Geometry check sheet. Reference: the model listing, model coordinates, mm. A direction names the side the tool comes from. Give positions to 0.01 mm unless a question says otherwise; leave off trailing zeros. Loops run counter-clockwise (first coordinate to the right, second up) from the corner with the lowest first, then second, coordinate; pieces in that order, holes last. Notation, with made-up numbers: (-31, 62) -> (-26, 62) arc R11 ccw to (-26, 72) -> close; hole circle Ø1 at (58, -30.75). An arc over 180 degrees is marked (long way). Write each question's results on one line, items separated by ' | '. Start each with the question number.
1) Set-up check for faces 1 (the face through (-33, 2, -5.1)), 2 (the face through (-41.133, 1.479, -1.286)), 3 (the face through (31, 2, 9)), 4 (the face through (19, 1, -6)), 5 (the face through (21, 1, 6)): record each of +Z, -Z, +X, -X, +Y, -Y from which the full face is reachable in a straight line by a thin tool's end or side.
2) Draft check along X on faces 6 (the face through (1, 0, -5)), 7 (the face through (-27.574, 1.521, -11.238)), 8 (the face through (17.5, 1.5, 5)), 9 (the face through (-41.5, 2, -7)). Enter one of: pulls with the +X half, pulls with the -X half, needs draft (parallel to the pull), parting line crosses it, or undercut.
3) Scan lines: line 1 (X direction, y = 1.6, z = 7); line 2 (Z direction, x = -32, y = 1.65); line 3 (Z direction, x = 0.5, y = 0.65). Record each from-to range of solid material in increasing order. Write a range as from..to.
4) Sectioned sample at C-C on y = 1.4. Count the separate pieces of the cut face and the enclosed holes in it, then the cut area to 3 significant figures.
5) Sectioned sample at A-A on x = 28.5. Record the cut outline in (y, z), then the cut area to 3 significant figures.
6) Sectioned sample at D-D on x = 1. Record the cut outline in (y, z).
7) Depth check by flat-ended pin: pin 1 (1 mm diameter, centred on x = -16, z = 3.5, fed in from -Y); pin 2 (0.9 mm diameter, centred on x = -18, y = 2, fed in from +Z); pin 3 (0.9 mm diameter, centred on y = 2, z = 7, fed in from +X); pin 4 (1.5 mm diameter, centred on x = -33.5, y = 2, fed in from +Z). Enter the tip coordinate at first touch or a pass-through.
```python
from build123d import *

# Parameters (mm, degrees)
SKETCH_1_W          = 83
SKETCH_1_H          = 12
EXTRUDE_1_DEPTH     = 3
SKETCH_2_W          = 10
SKETCH_2_H          = 3
EXTRUDE_2_DEPTH     = 3
SKETCH_3_R          = 1
CUT_EXTRUDE_1_DEPTH = 43.570529712
SKETCH_4_R          = 1.35
CUT_EXTRUDE_2_DEPTH = 43.570529712
CUT_EXTRUDE_3_DEPTH = 43.570529712
EXTRUDE_3_DEPTH     = 3
SKETCH_9_R          = 1.1
SKETCH_9_W          = 9
SKETCH_9_H          = 3.8
CUT_EXTRUDE_6_DEPTH = 44.900455579
SKETCH_8_R          = 4
CUT_EXTRUDE_5_DEPTH = 44.900455579
FILLET_1_R          = 8
FILLET_2_R          = 2
FILLET_3_R          = 1


with BuildPart() as part:
    # 草图1 → 凸台-拉伸1 (new body)
    with BuildSketch(Plane(origin=(0, 0, 0), x_dir=(1, 0, 0), z_dir=(0, 1, 0))):
        Rectangle(SKETCH_1_W, SKETCH_1_H)
    extrude(amount=EXTRUDE_1_DEPTH)

    # 草图2 → 凸台-拉伸2 (add)
    with BuildSketch(Plane(origin=(0, 3, 0), x_dir=(1, 0, 0), z_dir=(0, 1, 0))):
        with Locations((11.5, -7.5)):
            Rectangle(SKETCH_2_W, SKETCH_2_H)
        with Locations((-8.5, -7.5)):
            Rectangle(SKETCH_2_W, SKETCH_2_H)
        with Locations((31.5, -7.5)):
            Rectangle(SKETCH_2_W, SKETCH_2_H)
    extrude(amount=-EXTRUDE_2_DEPTH)

    # 草图3 → 切除-拉伸1 (cut, through all)
    with BuildSketch(Plane.XZ):
        with Locations((17.5, 6)):
            Circle(SKETCH_3_R)
        with Locations((5.5, 6)):
            Circle(SKETCH_3_R)
        with Locations((-2.5, 6)):
            Circle(SKETCH_3_R)
        with Locations((-14.5, 6)):
            Circle(SKETCH_3_R)
        with Locations((25.5, 6)):
            Circle(SKETCH_3_R)
        with Locations((37.5, 6)):
            Circle(SKETCH_3_R)
    extrude(amount=-CUT_EXTRUDE_1_DEPTH, mode=Mode.SUBTRACT)

    # 草图4 → 切除-拉伸2 (cut, through all)
    with BuildSketch(Plane(origin=(0, 3, 0), x_dir=(1, 0, 0), z_dir=(0, 1, 0))):
        with Locations(Location((28.5, 0, 0), (0, 0, 270))):
            Circle(SKETCH_4_R)
        with Locations(Location((36.5, 0, 0), (0, 0, 270))):
            Circle(SKETCH_4_R)
    extrude(amount=-CUT_EXTRUDE_2_DEPTH, mode=Mode.SUBTRACT)

    # 草图6 → 切除-拉伸3 (cut, through all)
    with BuildSketch(Plane(origin=(0, 3, 0), x_dir=(1, 0, 0), z_dir=(0, 1, 0))):
        Polygon((-41.5, 1), (-20.5, -6), (-41.5, -6), align=None)
    extrude(amount=-CUT_EXTRUDE_3_DEPTH, mode=Mode.SUBTRACT)

    # 草图5 → 凸台-拉伸3 (add)
    with BuildSketch(Plane(origin=(0, 3, 0), x_dir=(1, 0, 0), z_dir=(0, 1, 0))):
        Polygon((-41.5, 14), (-25.5, 14), (-1.5, 6), (-41.5, 6), align=None)
    extrude(amount=-EXTRUDE_3_DEPTH)

    # 草图9 → 切除-拉伸6 (cut, through all)
    with BuildSketch(Plane(origin=(0, 3, 0), x_dir=(1, 0, 0), z_dir=(0, 1, 0))):
        with Locations(Location((-38.5, 11, 0), (0, 0, 270))):
            Circle(SKETCH_9_R)
        with Locations(Location((-38.5, 3, 0), (0, 0, 270))):
            Circle(SKETCH_9_R)
        with Locations(Location((-26.5, 3, 0), (0, 0, 270))):
            Circle(SKETCH_9_R)
        with Locations(Location((-26.5, 11, 0), (0, 0, 270))):
            Circle(SKETCH_9_R)
        with Locations((-32.5, 7)):
            Rectangle(SKETCH_9_W, SKETCH_9_H)
    extrude(amount=-CUT_EXTRUDE_6_DEPTH, mode=Mode.SUBTRACT)

    # 草图8 → 切除-拉伸5 (cut, through all)
    with BuildSketch(Plane(origin=(0, 3, 0), x_dir=(1, 0, 0), z_dir=(0, 1, 0))):
        with Locations(Location((11, 0, 0), (0, 0, 270))):
            Circle(SKETCH_8_R)
        with Locations(Location((1, 0, 0), (0, 0, 270))):
            Circle(SKETCH_8_R)
        with Locations(Location((-9, 0, 0), (0, 0, 270))):
            Circle(SKETCH_8_R)
        with Locations(Location((-19, 0, 0), (0, 0, 270))):
            Circle(SKETCH_8_R)
        with Locations(Location((21, 0, 0), (0, 0, 270))):
            Circle(SKETCH_8_R)
    extrude(amount=-CUT_EXTRUDE_5_DEPTH, mode=Mode.SUBTRACT)

    # 圆角1
    fillet_1_edges = [part.edges().sort_by_distance(p)[0] for p in [
        (-20.5, 1.5, 6),
        (-25.5, 1.5, -14),
        (-1.5, 1.5, -6),
    ]]
    fillet(fillet_1_edges, radius=FILLET_1_R)

    # 圆角2
    fillet_2_edges = [part.edges().sort_by_distance(p)[0] for p in [
        (-41.5, 1.5, -1),
        (-41.5, 1.5, -14),
        (41.5, 1.5, 6),
        (41.5, 1.5, -6),
    ]]
    fillet(fillet_2_edges, radius=FILLET_2_R)

    # 圆角3
    fillet_3_edges = [part.edges().sort_by_distance(p)[0] for p in [
        (-28, 1.5, -8.9),
        (-28, 1.5, -5.1),
        (-37, 1.5, -5.1),
        (-37, 1.5, -8.9),
    ]]
    fillet(fillet_3_edges, radius=FILLET_3_R)


solid = part.part
```
Result:
1) face 1: +Y, -Y | face 2: +Z, -X, +Y, -Y | face 3: +Z, +X, -X, +Y, -Y | face 4: -Z, +X, +Y, -Y | face 5: +Z, +Y, -Y
2) face 6: needs draft | face 7: undercut | face 8: undercut | face 9: pulls with the -X half
3) line 1: -13.5..-3.5, 6.5..16.5, 26.5..36.5 | line 2: -14..-8.9, -5.1..2.17 | line 3: -6..-3.97, 3.97..6
4) separate pieces: 1 | enclosed holes: 12 | area: 913 mm^2
5) outline: (0, -6) -> (3, -6) -> (3, -1.35) -> (0, -1.35) -> close; (0, 1.35) -> (3, 1.35) -> (3, 9) -> (0, 9) -> close | area: 36.9 mm^2
6) outline: (0, -6) -> (3, -6) -> (3, -4) -> (0, -4) -> close; (0, 4) -> (3, 4) -> (3, 6) -> (0, 6) -> close
7) pin 1: y = 0 | pin 2: z = 6 | pin 3: x = 36.5 | pin 4: z = 1.92
